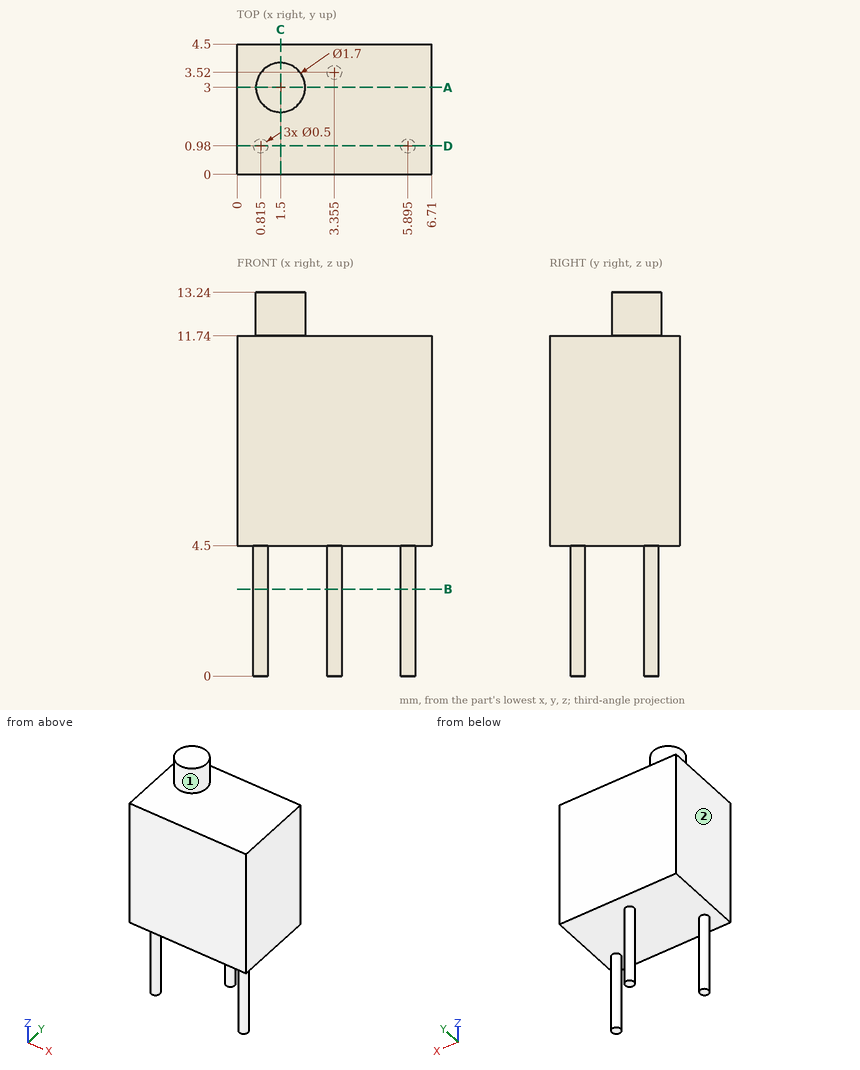
Verification items for this drawing (mm, ordinates from the low corner). A direction names the side the tool comes from. Coordinates: 2 decimals unless noted, no trailing zeros. Order: outer loops, then holes, each group sorted by start corner. A loop starts at its lowest first (then second) coordinate and runs counter-clockwise, first axis right, second up. Notation, with made-up numbers: M -40,59 L 3,59 A35 cw 3,94 Z; hole C -33,13.5 d5. An arc over 180 degrees is marked long. Use CSV: the item, a comma, the result in double quotes.
Item 1: Tool access check on the marked faces 1 and 2. Record the directions out of +Z, -Z, +X, -X, +Y, -Y that give a thin tool (end or side, any length) a straight path to the whole face; none if there is none.
Returned:
face 1,"+Z"
face 2,"+Z, -Z, -X, +Y, -Y"
Item 2: Cross-section at D-D on y = 0.98. Record the cut outline in (x, z) (3 decimals), then the cut area to 3 significant figures.
Returned:
outline,"M 0,4.5 L 0.565,4.5 L 0.565,0 L 1.065,0 L 1.065,4.5 L 5.645,4.5 L 5.645,0 L 6.145,0 L 6.145,4.5 L 6.71,4.5 L 6.71,11.74 L 0,11.74 Z"
area,"53.1 mm2"
Item 3: Cross-section at B-B on z = 3. Record the cut outline in (x, y) (3 decimals), then the cut area to 3 significant figures.
Returned:
outline,"C 0.815,0.98 d0.5; C 3.355,3.52 d0.5; C 5.895,0.98 d0.5"
area,"0.589 mm2"
Item 4: Cross-section at A-A on y = 3. Record the cut outline in (x, z), then the cut area to 3 significant figures.
Returned:
outline,"M 0,4.5 L 6.71,4.5 L 6.71,11.74 L 2.35,11.74 L 2.35,13.24 L 0.65,13.24 L 0.65,11.74 L 0,11.74 Z"
area,"51.1 mm2"
Item 5: Thickness scan on line 1 along Z through (x, y) = (1.5, 2.95); line 2 along Z through (x, y) = (6, 1.8); line 3 along X through (y, z) = (3.55, 3.75). Record the ranges inside material, lowest first.
Returned:
line 1,"z = 4.5 to 13.24"
line 2,"z = 4.5 to 11.74"
line 3,"x = 3.11 to 3.6"
Item 6: Cross-section at C-C on x = 1.5. Record the cut outline in (y, z).
Returned:
outline,"M 0,4.5 L 4.5,4.5 L 4.5,11.74 L 3.85,11.74 L 3.85,13.24 L 2.15,13.24 L 2.15,11.74 L 0,11.74 Z"
